Autodesk Inventor part; units mm, degrees
ref_plane "YZ Plane" through (0, 0, 0) normal (1, 0, 0) x (0, 1, 0)
ref_plane "XZ Plane" through (0, 0, 0) normal (0, 1, 0) x (-1, 0, 0)
ref_plane "XY Plane" through (0, 0, 0) normal (0, 0, 1) x (1, 0, 0)
sketch "Sketch1" plane through (0, 0, 0) normal (0, 1, 0) x (-1, 0, 0)
  line L0 (0, 0) -> (3.0089, 0) construction
  line L1 (3.0089, 0) -> (7.069, 5.8831) construction
  line L2 (7.069, 5.8831) -> (8.9606, 9.5326) construction
  line L3 (8.9606, 9.5326) -> (11.3861, 1.7338) construction
  line L4 (11.3861, 1.7338) -> (15.5604, 1.7338) construction
  spline S0 degree 4 poles (0, 0) (3.0089, 0) (7.069, 5.8831) (8.9606, 9.5326) (11.3861, 1.7338) (11.3861, 1.7338) (15.5604, 1.7338) knots 1 1 1 1 1 2 3 4 4 4 4 4
  line L5 (0, 0) -> (-2.509, 0)
  line L6 (-2.509, 0) -> (-2.509, 2.5)
  line L7 (-2.509, 2.5) -> (-1.0509, 2.5)
  line L8 (-1.0509, 2.5) -> (3.5176, 2.5) construction
  line L9 (3.5176, 2.5) -> (4.4785, 7.5024) construction
  line L10 (4.4785, 7.5024) -> (10.7757, 12.1884) construction
  line L11 (10.7757, 12.1884) -> (13.1491, 3.4753) construction
  line L12 (13.1491, 3.4753) -> (13.5495, 3.0077) construction
  line L13 (13.5495, 3.0077) -> (15.5604, 3.0077) construction
  spline S1 degree 4 poles (-1.0509, 2.5) (3.5176, 2.5) (4.4785, 7.5024) (10.7757, 12.1884) (13.1491, 3.4753) (13.5495, 3.0077) (15.5604, 3.0077) knots 1 1 1 1 1 2 3 4 4 4 4 4
  line L14 (15.5604, 3.0077) -> (15.5604, 1.7338)
  dimension "d0" = 2.5
extrude "Extrusion1" add sketch "Sketch1" along normal blind 8
sketch "Sketch2" plane through (1.0509, 0, 2.5) normal (0, 0, 1) x (1, 0, 0)
  circle A0 centre (-0.8088, 4) radius 1.45
  line L0 (-16.6113, 8) -> (0, 8)
  point P0 (-1.0509, 0)
  dimension "d3" = 2.9
  dimension "d14" = 4
extrude "Extrusion2" cut sketch "Sketch2" along normal mid plane 7
sketch "Sketch3" plane through (0, 0, 0) normal (0, -1, 0) x (1, 0, 0)
  line L0 (2.509, 0) -> (0, 0)
  line L1 (2.509, 2.5) -> (2.509, 0)
  line L2 (1.0509, 2.5) -> (2.509, 2.5)
  spline S0 degree 4 poles (-15.5604, 3.0077) (-13.5495, 3.0077) (-13.1491, 3.4753) (-10.7757, 12.1884) (-4.4785, 7.5024) (-3.5176, 2.5) (1.0509, 2.5) knots 0 0 0 0 0 0.333333 0.666667 1 1 1 1 1
  line L3 (-15.5604, 1.7338) -> (-15.5604, 3.0077)
  arc A0 (-7.1833, 8.351) -> (-19.9296, 12.3019) centre (-22.9296, -19.9129) ccw
  arc A1 (-10.767, 7.9081) -> (-19.9296, 10.3019) centre (-22.9296, -19.9129) ccw
  line L4 (-19.9296, 12.3019) -> (-19.9296, 10.3019)
  line L5 (-19.9296, 12.3019) -> (-25.9296, 12.3019)
  line L6 (-25.9296, 12.3019) -> (-25.9296, 10.3019)
  line L7 (-25.9296, 10.3019) -> (-19.9296, 10.3019)
  line L8 (-19.9296, 10.3019) -> (-19.9296, 12.3019)
  dimension "d6" = 6
  dimension "d7" = 2
extrude "Extrusion3" add sketch "Sketch3" against normal up to surface (8 mm away)
sketch "Sketch4" plane through (-25.9296, 0, 12.3019) normal (0, 0, 1) x (1, 0, 0)
  arc A0 (0.3271, 6.628) -> (0.3271, 0.742) centre (3.8271, 3.685) ccw
  arc A1 (26.9804, 2.7965) -> (26.9804, 5.2035) centre (26.1717, 4) ccw
  circle A2 centre (3.8592, 4) radius 2.5
  point P0 (25.9296, 0)
  dimension "d10" = 5
extrude "Extrusion4" cut sketch "Sketch4" against normal blind 10
fillet "Fillet1" radius 2 3 edges at (-25.9296, 0, 11.3019) (-25.9296, 8, 11.3019) (-10.767, 4, 7.9081)
properties part number "30_Cube_Chipadapter_Fluicis_clamp"
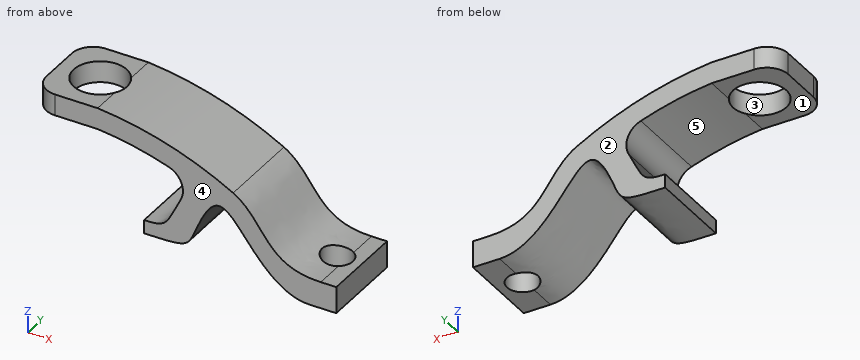
Source: CAD feature listing. Evaluate the final solid. Frame: model axes, mm. Face numbers are marked on the shaded views. A direction names the side the tool comes from. Round coordinates to 2 decimals unless told otherwise and drop trailing zeros.
1. Section query A-A on y = 4. Give the number of separate pieces and of enclosed holes in the cut face, and give its area (3 significant figures).
2. Ray query, L1, parallel to X at y = 4, z = 2.2; L2, parallel to Z at x = -23.5, y = 7; L3, parallel to Z at x = -12.75, y = 7.25. Return the intervals inside material, ascending.
3. Mould query, pull axis Y, two halves, no side actions, for the marked faces 1, 2 and 3. Classes: released by +Y, released by -Y, zero draft, split by the parting line, or undercut.
4. Access query for the marked faces 4 and 5. Directions: +Z, -Z, +X, -X, +Y, -Y. A direction counts if a zero-diameter tool reaches every point of the face in a straight line with its end or side. Return the directions, or none.
5. Contact query for flat-ended pins moving along their axis: pin 1 (4 mm diameter, centred on x = 0.24, y = 4, fed in from +Z); pin 2 (1 mm diameter, centred on x = -7.5, y = 5, fed in from +Z); pin 3 (0.7 mm diameter, centred on x = 1.5, y = 2.5, fed in from +Z); pin 4 (1.8 mm diameter, centred on x = -23.5, y = 4, fed in from -Z) (1 decimal). Output: stop coordinate, or through.
Answers below:
1. separate pieces: 3
1. enclosed holes: 0
1. area: 66.7 mm2
2. L1: x = -15.56 to -11.51, -4.2 to -1.21, 1.69 to 2.51
2. L2: z = 10.3 to 12.3
2. L3: z = 1.8 to 4.82, 8.61 to 10.8
3. face 1: zero draft
3. face 2: released by +Y
3. face 3: undercut
4. face 4: +Z, -Z, +X, -X, -Y
4. face 5: -X, +Y, -Y
5. pin 1: stops at z = 3
5. pin 2: stops at z = 8.79
5. pin 3: stops at z = 2.5
5. pin 4: passes through
